from build123d import *

# Parameters (mm, degrees)
SKETCH1_R           = 3.175
BOSS_EXTRUDE1_DEPTH = 3.175


with BuildPart() as part:
    # Sketch1 → Boss-Extrude1 (new body)
    with BuildSketch(Plane.XY.offset(50.8)):
        with BuildLine():
            Line((101.6, 15.875), (0, 25.4))
            Line((0, 25.4), (-12.7, 25.4))
            Line((-12.7, 25.4), (-12.7, -25.4))
            Line((-12.7, -25.4), (0, -25.4))
            Line((0, -25.4), (101.6, -15.875))
            ThreePointArc((101.6, -15.875), (117.475, 0), (101.6, 15.875))
        make_face()
        with Locations((101.6, 0)):
            Circle(SKETCH1_R, mode=Mode.SUBTRACT)
    extrude(amount=BOSS_EXTRUDE1_DEPTH)


solid = part.part
The model under review builds one solid part; all positions refer to its coordinate system, in mm. Coordinates: 2 decimals unless noted, no trailing zeros. Loops run counter-clockwise (first coordinate to the right, second up) from the corner with the lowest first, then second, coordinate; pieces in that order, holes last. Notation, with made-up numbers: M 75,1 L 131,1 A22 ccw 131,10 Z; hole C 36,-38.5 d1. An arc over 180 degrees is marked long. Put each result on its own line as item: value. Start each with the question number.
Q1. Add section C-C (x = 56). Write out the cut boundary in (y, z) (3 decimals).
Q2. Add section D-D (y = 9.5). Write out the cut boundary in (x, z) (3 decimals), and give its area (3 significant figures).
Q3. Wall thickness on line 1 (Y direction, x = 101.6, z = 52.15) (3 decimals); line 2 (X direction, y = 1.5, z = 52.6); line 3 (X direction, y = -4, z = 52.9): over which ranges is each line inside the solid? List them lowest first.
Q4. Add section B-B (z = 53.2). Write out the cut boundary in (x, y) (3 decimals), and give its area (3 significant figures).
Q5. Add section A-A (y = 0). Write out the cut boundary in (x, z) (3 decimals), and give its area (3 significant figures).
Q6. Clearance check with a flat-ended pin moving along its axis: pin 1 (5 mm diameter, centred on x = 101.6, y = 0, fed in from -Z). State where the tip first meets the part, or that it passes through.
Answers:
1. outline: M -20.15,50.8 L 20.15,50.8 L 20.15,53.975 L -20.15,53.975 Z
2. outline: M -12.7,50.8 L 114.319,50.8 L 114.319,53.975 L -12.7,53.975 Z
2. area: 403 mm^2
3. line 1: y = -15.875 to -3.175, 3.175 to 15.875
3. line 2: x = -12.7 to 98.8, 104.4 to 117.4
3. line 3: x = -12.7 to 116.96
4. outline: M -12.7,-25.4 L 0,-25.4 L 101.6,-15.875 A15.875 ccw 101.6,15.875 L 0,25.4 L -12.7,25.4 Z; hole C 101.6,0 d6.35
4. area: 5,200 mm^2
5. outline: M -12.7,50.8 L 98.425,50.8 L 98.425,53.975 L -12.7,53.975 Z; M 104.775,50.8 L 117.475,50.8 L 117.475,53.975 L 104.775,53.975 Z
5. area: 393 mm^2
6. pin 1: passes through
